Verification items for the finished model (mm, model axes). Round coordinates to 2 decimals unless told otherwise and drop trailing zeros. Write each loop counter-clockwise with the first axis right and the second up, starting at its lowest first coordinate (ties: lowest second). Pieces come first, ordered by that corner, then holes. Notation, with made-up numbers: M 75,41 L 110,41 A30 ccw 110,65 Z; hole C 12,-34 d1. An arc over 180 degrees is marked long. One line per question, with ' | ' between items. Start each with the question number.
Q1. Cross-section at B-B (z = 0). Record the boundary of the cut face in (x, y) (3 decimals).
Q2. Cross-section at C-C (x = 4.4). Record the boundary of the cut face in (y, z), then the cut area to 3 significant figures.
Q3. Gauge pin test, flat end, axial feed: pin 1 (1 mm diameter, centred on x = 0.5, y = -0.5, fed in from +Z). Record the tip position at first contact, or that the pin passes through.
Q4. Thickness scan on line 1 along Y through (x, z) = (0.7, 0.3); line 2 along Z through (x, y) = (5.35, -0.1); line 3 along Z through (x, y) = (5.5, -1). Record the ranges inside material, lowest first. Write a range as from..to.
Q5. Release check for a two-part mould opening along Z. For faces 1 (the face through (0, 1.2, 0)), 2 (the face through (0.83, 0, 0)), 3 (the face through (3.8, -1.5, -0.07)) record: released by +Z, released by -Z, zero draft, split by the parting line, or undercut.
Q6. Cross-section at A-A (y = 0). Record the boundary of the cut face in (x, z) (3 decimals), then the cut area to 3 significant figures.
Autodesk Inventor part; units mm, degrees
ref_plane "YZ Plane" through (0, 0, 0) normal (1, 0, 0) x (0, 1, 0)
ref_plane "XZ Plane" through (0, 0, 0) normal (0, 1, 0) x (-1, 0, 0)
ref_plane "XY Plane" through (0, 0, 0) normal (0, 0, 1) x (1, 0, 0)
sketch "Sketch1" plane through (0, 0, 0) normal (0, 0, 1) x (1, 0, 0)
  line L0 (0, 0) -> (6, 0)
  line L1 (6, 0) -> (6, 1.5)
  line L2 (6, 1.5) -> (2.35, 1.5)
  line L3 (2.35, 1.5) -> (2.15, 1.5)
  line L4 (2.15, 1.5) -> (1.67, 1.5)
  line L5 (1.65, 1.515) -> (1.65, 1.515)
  line L6 (1.65, 1.515) -> (0.415, 2.75)
  line L7 (0.415, 2.75) -> (0, 2.75)
  line L8 (0, 2.75) -> (0, 0)
  line L9 (1.65, 1.515) -> (1.65, 1.52)
  arc A0 (1.65, 1.52) -> (1.67, 1.5) centre (1.67, 1.52) ccw
  dimension "d17" = 6
  dimension "d18" = 0.415
  dimension "d19" = 1.65
  dimension "d20" = 0
  dimension "d21" = 5.5
  dimension "d22" = 3
  dimension "d23" = 3
  dimension "d25" = 45
  dimension "d26" = 0.2
  dimension "d28" = 0.02
  dimension "d29" = 3.65
  dimension "d30" = 0.02
  dimension "d52" = 0.7
revolve "Revolution1" add sketch "Sketch1" angle 360 about axis through (0, 0, 0) along (1, 0, 0)
thread "Thread1"
sketch "Sketch2" plane through (0, 0, 0) normal (-1, 0, 0) x (0, 0, 1)
  circle A0 centre (0, 0) radius 1.4 construction
  circle A1 centre (0, 0) radius 0.98 construction
  line L0 (0, 0) -> (0.8487, 0.49)
  line L1 (0, 0) -> (0.98, 0) construction
  line L2 (0, 0) -> (0.8487, -0.49)
  line L3 (0, 0) -> (0.98, 0) construction
  line L4 (0.8487, 0.49) -> (1.4, 0)
  line L5 (1.4, 0) -> (0.8487, -0.49)
  dimension "d34" = 2.8
  dimension "d35" = 1.96
  dimension "d39" = 30
  dimension "d40" = 330
extrude "Extrusion1" cut sketch "Sketch2" against normal blind 0.83
pattern_circular "Circular Pattern1" count 6 over 360 about axis through (-10, 0, 0) along (1, 0, 0) of "Extrusion1"
fillet "Fillet1" radius 0.3 12 edges at (0.415, 0.49, 0.8487) (0.415, 0, 1.4) (0.415, -0.49, 0.8487) (0.415, -0.98, 0) (0.415, -1.2124, 0.7) (0.415, -1.2124, -0.7) (0.415, -0.49, -0.8487) (0.415, 0, -1.4) (0.415, 0.49, -0.8487) (0.415, 1.2124, -0.7) (0.415, 0.98, 0) (0.415, 1.2124, 0.7)
equation "\"d17\" = l_"
equation "\"d18\" = 0.5 * t"
equation "\"d19\" = k"
equation "\"d21\" = dk"
equation "\"d22\" = d"
equation "\"d23\" = ds_"
equation "\"d25\" = 0.5 * headAngle"
equation "\"d26\" = x"
equation "\"d28\" = r"
equation "\"d29\" = b"
equation "\"d32\" = b"
equation "\"d34\" = A_"
equation "\"d35\" = 0.7 * A_"
equation "\"d43\" = t"
equation "\"d48\" = v"
equation "\"A_\" = 2.8"
equation "\"t\" = 0.83"
equation "\"v\" = 0.1 * d"
equation "\"dk\" = 5.5"
equation "\"k\" = 1.65"
equation "\"l_\" = 6"
equation "\"shldr\" = 0"
equation "\"d\" = 3"
equation "\"p\" = 0.8"
equation "\"x\" = 0.2"
equation "\"ds_\" = 3"
equation "\"headAngle\" = 90deg"
equation "\"c_\" = 0.35 * v"
equation "\"r\" = 0.02"
properties part number "Hexalobular socket countersunk flat head screw ISO 14581 - M3x6-4.8" material "Steel"
Determined:
1) outline: M 0,-2.75 L 0.415,-2.75 L 1.65,-1.515 A0.02 cw 1.67,-1.5 L 6,-1.5 L 6,1.5 L 1.67,1.5 A0.02 cw 1.651,1.515 L 0.415,2.75 L 0,2.75 L 0,0.996 L 0.83,0.996 L 0.83,-0.996 L 0,-0.996 Z
2) outline: C 0,0 d3 | area: 7.07 mm²
3) pin 1: stops at z = 2.75
4) line 1: y = -2.45..-1.08, 1.08..2.45 | line 2: z = -1.5..1.5 | line 3: z = -1.12..1.12
5) face 1: zero draft | face 2: undercut | face 3: split by the parting line
6) outline: M 0,-2.75 L 0.415,-2.75 L 1.65,-1.515 A0.02 cw 1.67,-1.5 L 6,-1.5 L 6,1.5 L 1.67,1.5 A0.02 cw 1.651,1.515 L 0.415,2.75 L 0,2.75 L 0,1.248 L 0.83,1.248 L 0.83,-1.248 L 0,-1.248 Z | area: 18.5 mm²
